For this review, take the finished solid that the model builds, in its own axes (mm). A direction names the side the tool comes from. Coordinates: 2 decimals unless noted, no trailing zeros. Order: outer loops, then holes, each group sorted by start corner. A loop starts at its lowest first (then second) coordinate and runs counter-clockwise, first axis right, second up. Notation, with made-up numbers: (-6.75, 37) -> (-2.75, 37) arc R13 ccw to (-2.75, 57) -> close; hole circle Ø9 at (21.25, 24.5). An arc over 180 degrees is marked (long way). Return JSON: item names as keys, results as strings. Group by question number.
Item 1: Take a section at D-D (x = 5.5). Write out the cut boundary in (y, z), then the cut area to 3 significant figures.
Item 2: Draft analysis for pull direction X (two halves, no side actions). For faces 1 (the cylindrical face through (-7.75, 0.78, -1.72)), 2 (the flat face through (-11.112, 4, -15)), 3 (the cylindrical face through (9.68, 4.109, -22.454)), 4 (the flat face through (-0.2, 0, 8.2)), state which applies: +X half, -X half, draft (parallel to the pull), parting line (faces both ways), or undercut.
Item 3: Take a section at C-C (y = 4). Count the separate pieces of the cut face and the enclosed holes in it, then the cut area to 3 significant figures.
Item 4: Insertion check: pin 1 (10 mm diameter, centred on x = 2, z = -13, fed in from +Y); pin 2 (12 mm diameter, centred on x = -5, z = 0, fed in from +Y). Each pin has a flat end and moves straight along its axis. Give the tip position at first contact, or say it passes through.
Item 5: Take a section at B-B (x = 0). Write out the cut boundary in (y, z), then the cut area to 3 significant figures.
Item 6: For line 1 along X through (y, z) = (2.5, -19.05); line 2 along X through (y, z) = (5, -20.5); line 3 along Y through (x, z) = (-4.5, 13), list the stretches that pass through material, from the lowest coordinate up.
Item 7: Take a section at A-A (z = 0). Write out the cut boundary in (x, y), then the cut area to 3 significant figures.
Item 8: Machinability: for faces 5 (the cylindrical face through (-9.754, 4.109, -22.38)), 6 (the cylindrical face through (4.203, 4.109, -23.467)), 7 (the cylindrical face through (-0.157, 4.914, -15.505)), which of the approach directions +Z, -Z, +X, -X, +Y, -Y give a long, thin tool a straight path to every point of the face, cutting with its end or side? Answer none if there is none.
```python
from build123d import *

# Parameters (mm, degrees)
SKETCH1_R           = 7.9375
BOSS_EXTRUDE1_DEPTH = 1.5875
SKETCH2_R           = 2.38125
BOSS_EXTRUDE2_DEPTH = 8.334375
CUT_EXTRUDE1_START  = -6.746875
CUT_EXTRUDE1_DEPTH  = 6.746875


with BuildPart() as part:
    # Sketch1 → Boss-Extrude1 (new body)
    with BuildSketch(Plane(origin=(0, 0, 0), x_dir=(1, 0, 0), z_dir=(0, 1, 0))):
        with BuildLine():
            Line((-14.3002, -24.3332), (-9.271, -28.0416))
            Line((-9.271, -28.0416), (9.271, -28.0416))
            Line((9.271, -28.0416), (14.3002, -24.3332))
            Line((14.3002, -24.3332), (14.3002, 5.9944))
            ThreePointArc((14.3002, 5.9944), (0, 15.505758653), (-14.3002, 5.9944))
            Line((-14.3002, 5.9944), (-14.3002, -24.3332))
        make_face()
        with Locations(Location((0, 0, 0), (0, 0, 270))):
            Circle(SKETCH1_R, mode=Mode.SUBTRACT)
    extrude(amount=BOSS_EXTRUDE1_DEPTH)

    # Sketch2 → Boss-Extrude2 (add)
    with BuildSketch(Plane.XZ):
        with BuildLine():
            Line((-11.1125, -12.601058837), (-11.1125, -19.05))
            ThreePointArc((-11.1125, -19.05), (-9.717596045, -22.417596045), (-6.35, -23.8125))
            Line((-6.35, -23.8125), (-5.983425441, -23.8125))
            ThreePointArc((-5.983425441, -23.8125), (-4.22646321, -23.476566386), (-2.717363519, -22.516157205))
            ThreePointArc((-2.717363519, -22.516157205), (0, -21.4376), (2.717363519, -22.516157205))
            ThreePointArc((2.717363519, -22.516157205), (4.22646321, -23.476566386), (5.983425441, -23.8125))
            Line((5.983425441, -23.8125), (6.35, -23.8125))
            ThreePointArc((6.35, -23.8125), (9.717596045, -22.417596045), (11.1125, -19.05))
            Line((11.1125, -19.05), (11.1125, -12.601058837))
            ThreePointArc((11.1125, -12.601058837), (11.377973728, -11.033206497), (12.144798566, -9.640146223))
            ThreePointArc((12.144798566, -9.640146223), (0, -15.505758653), (-12.144798566, -9.640146223))
            ThreePointArc((-12.144798566, -9.640146223), (-11.377973728, -11.033206497), (-11.1125, -12.601058837))
        make_face()
        with Locations(Location((-6.35, -19.05, 0), (0, 0, 270))):
            Circle(SKETCH2_R, mode=Mode.SUBTRACT)
        with Locations(Location((6.35, -19.05, 0), (0, 0, 270))):
            Circle(SKETCH2_R, mode=Mode.SUBTRACT)
    extrude(amount=-BOSS_EXTRUDE2_DEPTH)

    # Sketch3 → Cut-Extrude1 (cut)
    with BuildSketch(Plane(origin=(0, 8.334375, 0), x_dir=(1, 0, 0), z_dir=(0, 1, 0)).offset(CUT_EXTRUDE1_START)):
        with BuildLine():
            Line((-11.1125, 19.05), (-11.1125, 11.999376898))
            ThreePointArc((-11.1125, 11.999376898), (-10.813271374, 11.536258648), (-10.268096404, 11.618724011))
            ThreePointArc((-10.268096404, 11.618724011), (0, 15.505758653), (10.268096404, 11.618724011))
            ThreePointArc((10.268096404, 11.618724011), (10.813271374, 11.536258648), (11.1125, 11.999376898))
            Line((11.1125, 11.999376898), (11.1125, 19.05))
            Line((11.1125, 19.05), (16.416178114, 6.350325815))
            Line((16.416178114, 6.350325815), (-16.620971452, 6.890442702))
            Line((-16.620971452, 6.890442702), (-11.1125, 19.05))
        make_face()
    extrude(amount=CUT_EXTRUDE1_DEPTH, mode=Mode.SUBTRACT)


solid = part.part
```
Findings below:
{
 "1": {"outline": "(0, -23.79) -> (8.33, -23.79) -> (8.33, -21.27) -> (0, -21.27) -> close; (0, -16.83) -> (8.33, -16.83) -> (8.33, -14.5) -> (1.59, -14.5) -> (1.59, -5.72) -> (0, -5.72) -> close; (0, 5.72) -> (1.59, 5.72) -> (1.59, 28.04) -> (0, 28.04) -> close", "area": "89.7 mm2"},
 "2": {"face 1": "undercut", "face 2": "-X half", "face 3": "+X half", "face 4": "draft"},
 "3": {"separate pieces": "1", "enclosed holes": "2", "area": "157 mm2"},
 "4": {"pin 1": "stops at y = 8.33", "pin 2": "stops at y = 1.59"},
 "5": {"outline": "(0, -21.44) -> (8.33, -21.44) -> (8.33, -15.51) -> (1.59, -15.51) -> (1.59, -7.94) -> (0, -7.94) -> close; (0, 7.94) -> (1.59, 7.94) -> (1.59, 28.04) -> (0, 28.04) -> close", "area": "93.4 mm2"},
 "6": {"line 1": "x = -11.11 to -8.73, -3.97 to 3.97, 8.73 to 11.11", "line 2": "x = -10.89 to -8.24, -4.46 to 4.46, 8.24 to 10.89", "line 3": "y = 0 to 1.59"},
 "7": {"outline": "(-14.3, 0) -> (-7.94, 0) -> (-7.94, 1.59) -> (-14.3, 1.59) -> close; (7.94, 0) -> (14.3, 0) -> (14.3, 1.59) -> (7.94, 1.59) -> close", "area": "20.2 mm2"},
 "8": {"face 5": "-Z, -X, +Y, -Y", "face 6": "-Z, +Y, -Y", "face 7": "+Z, +Y"}
}
